Work out the finished part from the listing and answer in its coordinate system (mm). A direction names the side the tool comes from. Round coordinates to 2 decimals unless told otherwise and drop trailing zeros. Loops run counter-clockwise (first coordinate to the right, second up) from the corner with the lowest first, then second, coordinate; pieces in that order, holes last.
```python
from build123d import *

# Parameters (mm, degrees)
F0_R      = 12.7
F1_DEPTH  = 59.69
F2_W      = 30.988
F2_H      = 30.988
F3_DEPTH  = 16.6624
F7_DEPTH  = 21.971
F9_DEPTH  = 21.971
F10_R     = 14.986
F11_DEPTH = 22.86
F12_W     = 11.938
F12_H     = 5.08
F13_DEPTH = 118.6444


with BuildPart() as f1:
    # F0 (on Right) → F1 (new body, symmetric)
    with BuildSketch(Plane.YZ):
        Circle(F0_R)
    extrude(amount=F1_DEPTH, both=True)

    # F2 (on Right) → F3 (join, symmetric)
    with BuildSketch(Plane.YZ):
        Rectangle(F2_W, F2_H)
    extrude(amount=F3_DEPTH, both=True)

    # F6 (on offset) → F7 (join)
    with BuildSketch(Plane.YZ.offset(36.9824)):
        Polygon((-20.32, 5.969), (-20.32, -11.557), (-15.0749, -11.557), (-15.0749, -38.712503105), (0, -38.712503105), (15.0749, -38.712503105), (15.0749, -11.557), (20.32, -11.557), (20.32, 5.969), (17.145, 5.969), (6.731, 16.837296895), (0, 16.837296895), (-6.731, 16.837296895), (-17.145, 5.969), align=None)
    extrude(amount=F7_DEPTH)

    # F8 (on offset) → F9 (join)
    with BuildSketch(Plane(origin=(-33.6804, 0, 0), x_dir=(0, -1, 0), z_dir=(-1, 0, 0))):
        Polygon((-15.0749, -38.712503105), (15.0749, -38.712503105), (15.0749, -11.557), (20.32, -11.557), (20.32, 5.969), (17.145, 5.969), (6.731, 16.837296895), (-6.731, 16.837296895), (-17.145, 5.969), (-20.32, 5.969), (-20.32, -11.557), (-15.0749, -11.557), align=None)
    extrude(amount=F9_DEPTH)

    # F10 (on face) → F11 (join)
    with BuildSketch(Plane(origin=(0, 15.494, 0), x_dir=(-1, 0, 0), z_dir=(0, 1, 0))):
        Circle(F10_R)
    extrude(amount=F11_DEPTH)

    # F12 (on face) → F13 (cut, through all)
    with BuildSketch(Plane.YZ.offset(58.9534)):
        with Locations((0, -38.712503105)):
            Rectangle(F12_W, F12_H)
    extrude(amount=-F13_DEPTH, mode=Mode.SUBTRACT)


solid = f1.part
```
1. Given pin 1 (10 mm diameter, centred on y = 32.5, z = 11, fed in from -X); pin 2 (11 mm diameter, centred on x = 46.5, z = -18.5, fed in from -Y); pin 3 (2 mm diameter, centred on x = 33.5, z = -9, fed in from +Y), each flat-ended and moving along its own axis, determine where each tip first touches the part or whether it passes through.
Answer key:
pin 1: stops at x = -13.73
pin 2: stops at y = -15.07
pin 3: stops at y = 9.86
2. Find section B-B (y = 0). Write down the section's boundary in (x, z), then the cut area to 3 significant figures.
Answer key:
outline: (-59.69, -12.7) - (-55.65, -12.7) - (-55.65, -36.17) - (-33.68, -36.17) - (-33.68, -12.7) - (-16.66, -12.7) - (-16.66, -15.49) - (16.66, -15.49) - (16.66, -12.7) - (36.98, -12.7) - (36.98, -36.17) - (58.95, -36.17) - (58.95, -12.7) - (59.69, -12.7) - (59.69, 12.7) - (58.95, 12.7) - (58.95, 16.84) - (36.98, 16.84) - (36.98, 12.7) - (16.66, 12.7) - (16.66, 15.49) - (-16.66, 15.49) - (-16.66, 12.7) - (-33.68, 12.7) - (-33.68, 16.84) - (-55.65, 16.84) - (-55.65, 12.7) - (-59.69, 12.7) - close
area: 4,430 mm2
3. Consider probe 1 along X at (y, z) = (-17, -5); probe 2 along Y at (x, z) = (-51, -10.5); probe 3 along Y at (x, z) = (-11, -10.5). Determine where each line is inside the solid, lowest interval first.
Answer key:
probe 1: x = -55.65 to -33.68, 36.98 to 58.95
probe 2: y = -20.32 to 20.32
probe 3: y = -15.49 to 15.49
4. Determine the mould class of faces 5 (the face through (-45, 11, -38.713)), 6 (the face through (16.662, -7, 11)), 7 (the face through (59.69, 0, 0)) for opening direction X: +X half, -X half, draft (parallel to the pull), parting line (faces both ways), or undercut.
Answer key:
face 5: draft
face 6: undercut
face 7: +X half
5. Find section C-C (x = 0). Write down the section's boundary in (y, z).
Answer key:
outline: (-15.49, -15.49) - (15.49, -15.49) - (15.49, -14.99) - (38.35, -14.99) - (38.35, 14.99) - (15.49, 14.99) - (15.49, 15.49) - (-15.49, 15.49) - close
6. Which of the six approach directions +Z, -Z, +X, -X, +Y, -Y give full straight-line access (tool end or side, diameter ignored) to faces 1 (the face through (0, 0, -15.494)), 2 (the face through (-57.64, -2.75, -12.4)), 3 (the face through (1.95, 26.76, 14.86)), 4 (the face through (48, 20.32, -3))?
Answer key:
face 1: -Z, +Y, -Y
face 2: -X
face 3: +Y
face 4: +Z, -Z, +X, +Y
